Geometry check sheet. Reference: the model listing, model coordinates, mm. Face numbers are marked on the shaded views. Round coordinates to 2 decimals unless told otherwise and drop trailing zeros. Loops run counter-clockwise (first coordinate to the right, second up) from the corner with the lowest first, then second, coordinate; pieces in that order, holes last.
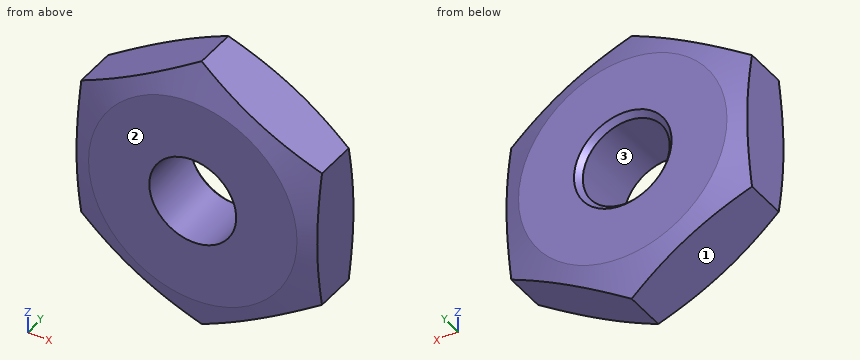
```python
from build123d import *

# Parameters (mm, degrees)
EXTRUDE_1_DEPTH       = 10
M14X1_5_1_D           = 12.5
M14X1_5_1_CSINK_D     = 14.05
M14X1_5_1_CSINK_ANGLE = 90


with BuildPart() as part:
    # 草图1 → 凸台-拉伸1 (new body)
    with BuildSketch(Plane(origin=(0, 0, 0), x_dir=(1, 0, 0), z_dir=(0, 1, 0))):
        Polygon((0, -20), (17.320508076, -10), (17.320508076, 10), (0, 20), (-17.320508076, 10), (-17.320508076, -10), align=None)
    extrude(amount=EXTRUDE_1_DEPTH)

    # M14x1.5 螺纹孔1 (through all)
    with Locations(Plane(origin=(0, 10, 0), x_dir=(1, 0, 0), z_dir=(0, 1, 0))):
        with Locations((0, 0)):
            CounterSinkHole(M14X1_5_1_D / 2, M14X1_5_1_CSINK_D / 2, counter_sink_angle=M14X1_5_1_CSINK_ANGLE)

    # 草图7 → 切除-旋转1 (revolve, cut)
    with BuildSketch(Plane(origin=(0, 0, 0), x_dir=(0, 0, -1), z_dir=(1, 0, 0))):
        Polygon((20, 10), (20, 8), (15, 10), align=None)
        Polygon((20, 2), (15, 0), (20, 0), align=None)
    revolve(axis=Axis((0, 15.71595543, 0), (0, -1, 0)), mode=Mode.SUBTRACT)


solid = part.part
```
1) Gauge pin test, flat ends, axial feed: pin 1 (2 mm diameter, centred on y = 7, z = -12, fed in from -X); pin 2 (3 mm diameter, centred on x = 1, y = 5, fed in from +Z); pin 3 (1 mm diameter, centred on x = -10.5, y = 4.5, fed in from -Z). Record the tip position at first contact, or that the pin passes through.
Report:
pin 1: stops at x = -15.59
pin 2: stops at z = 20
pin 3: stops at z = -14.23
2) Sectioned sample at A-A, the plane y = 6.25. Record the cut outline in (x, z), then the cut area to 3 significant figures.
Report:
outline: (-17.32, -10) - (0, -20) - (17.32, -10) - (17.32, 10) - (0, 20) - (-17.32, 10) - close; hole circle Ø12.5 at (0, 0)
area: 917 mm2
3) Scan lines: line 1 along Z through (x, y) = (0, 7.25); line 2 along Z through (x, y) = (4.5, 5.25); line 3 along Z through (x, y) = (-9, 5). Record each from-to range of solid material in increasing order.
Report:
line 1: z = -20 to -6.25, 6.25 to 20
line 2: z = -17.4 to -4.34, 4.34 to 17.4
line 3: z = -14.8 to 14.8
4) Mould release check, pull along Z, two halves, no side actions. Record for the marked faces 1, 2 and 3: +Z half, -Z half, draft (parallel to the pull), parting line (faces both ways), or undercut.
Report:
face 1: -Z half
face 2: draft
face 3: undercut
